The listing builds one solid part. Answer for the finished solid, in the listing's coordinates (mm). Face numbers are marked on the shaded views. A direction names the side the tool comes from. Coordinates: 2 decimals unless noted, no trailing zeros. Write each loop counter-clockwise with the first axis right and the second up, starting at its lowest first coordinate (ties: lowest second). Pieces come first, ordered by that corner, then holes. Notation, with made-up numbers: M 80.5,-17.75 L 112.5,-17.75 A21 ccw 112.5,-1.75 Z; hole C 2,2 d2. An arc over 180 degrees is marked long. Write item = value, one per line. Start each with the question number.
```python
from build123d import *

# Parameters (mm, degrees)
SKETCH2_W           = 20
SKETCH2_H           = 5
BOSS_EXTRUDE1_DEPTH = 7.2
CUT_EXTRUDE1_REACH  = 23.403
SKETCH3_W           = 3.2
SKETCH3_H           = 3
CHAMFER1_SIZE       = 0.5


with BuildPart() as part:
    # Sketch2 → Boss-Extrude1 (new body)
    with BuildSketch(Plane.XY):
        Rectangle(SKETCH2_W, SKETCH2_H)
    extrude(amount=BOSS_EXTRUDE1_DEPTH)

    # Sketch3 → Cut-Extrude1 (cut, up to next)
    with BuildSketch(Plane(origin=(10, 0, 0), x_dir=(0, 0, -1), z_dir=(1, 0, 0)), mode=Mode.PRIVATE) as cut_extrude1_sk1:
        with Locations((-3.6, -1)):
            Rectangle(SKETCH3_W, SKETCH3_H)
    cut_extrude1_tool1 = extrude(cut_extrude1_sk1.sketch, amount=-CUT_EXTRUDE1_REACH, mode=Mode.PRIVATE) & part.part
    add(cut_extrude1_tool1.solids().sort_by_distance((10, -1, 3.6))[0], mode=Mode.SUBTRACT)

    # Chamfer1
    chamfer1_edges = [part.edges().sort_by_distance(p)[0] for p in [
        (0, 2.5, 0),
        (0, 2.5, 7.2),
    ]]
    chamfer(chamfer1_edges, length=CHAMFER1_SIZE)


solid = part.part
```
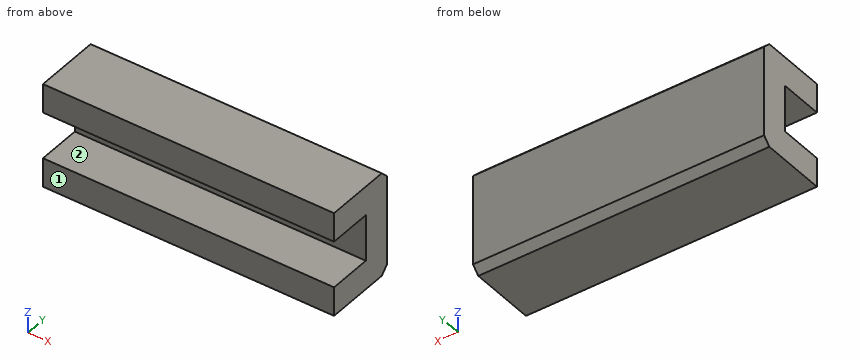
1. For the marked faces 1 and 2, determine the directions among +Z, -Z, +X, -X, +Y, -Y from which every point of the face is accessible in a straight line to the end or side of a thin tool.
2. Straight lines are drawn through the part: L1, parallel to Z at x = 6.25, y = 0.1; L2, parallel to Y at x = -5, z = 2.5; L3, parallel to Z at x = -8.5, y = 2.15. For each, find the intervals that lie inside material, in ascending order. Write a range as [from, to].
3. The part is cut by section C-C, the plane z = 3.25. Write down the section's boundary in (x, y).
4. The part is cut by section B-B, the plane x = -1. Write down the section's boundary in (y, z), and give its area (4 significant figures).
5. The part is cut by section A-A, the plane y = 0. Write down the section's boundary in (x, z).
Solution:
q1.face_1 = +Z, -Z, +X, -X, -Y
q1.face_2 = +X, -X, -Y
q2.L1 = [0, 2], [5.2, 7.2]
q2.L2 = [0.5, 2.5]
q2.L3 = [0.15, 7.05]
q3.outline = M -10,0.5 L 10,0.5 L 10,2.5 L -10,2.5 Z
q4.outline = M -2.5,0 L 2,0 L 2.5,0.5 L 2.5,6.7 L 2,7.2 L -2.5,7.2 L -2.5,5.2 L 0.5,5.2 L 0.5,2 L -2.5,2 Z
q4.area = 26.15 mm^2
q5.outline = M -10,0 L 10,0 L 10,2 L -10,2 Z; M -10,5.2 L 10,5.2 L 10,7.2 L -10,7.2 Z
